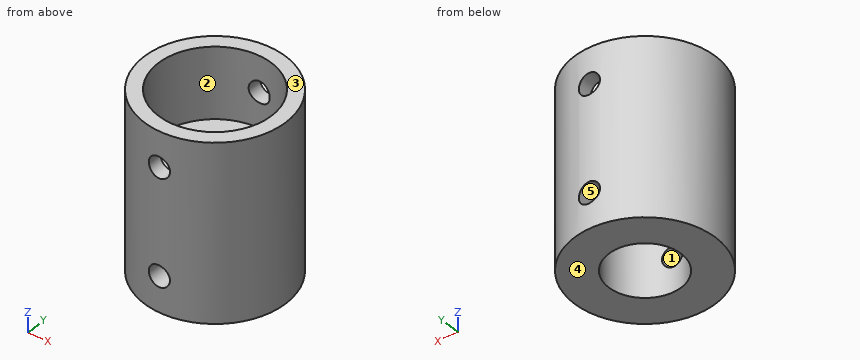
from build123d import *

# Parameters (mm, degrees)
ESQUISSE1_R                  = 20
ESQUISSE1_R_2                = 10.25
BOSS_EXTRU_1_DEPTH           = 50
ESQUISSE2_R                  = 16
ENL_V_MAT_EXTRU_1_DEPTH      = 20
ESQUISSE3_R                  = 3
ENL_V_MAT_EXTRU_2_DEPTH      = 21
ENL_V_MAT_EXTRU_2_DEPTH_BACK = 21


with BuildPart() as part:
    # Esquisse1 → Boss.-Extru.1 (new body)
    with BuildSketch(Plane.XY):
        Circle(ESQUISSE1_R)
        Circle(ESQUISSE1_R_2, mode=Mode.SUBTRACT)
    extrude(amount=BOSS_EXTRU_1_DEPTH)

    # Esquisse2 → Enlèv. mat.-Extru.1 (cut)
    with BuildSketch(Plane.XY.offset(50)):
        Circle(ESQUISSE2_R)
    extrude(amount=-ENL_V_MAT_EXTRU_1_DEPTH, mode=Mode.SUBTRACT)

    # Esquisse3 → Enlèv. mat.-Extru.2 (cut, two sides)
    with BuildSketch(Plane(origin=(0, 0, 0), x_dir=(1, 0, 0), z_dir=(0, 1, 0))) as enl_v_mat_extru_2_sk:
        with Locations(Location((0, -10, 0), (0, 0, 270))):  # turned: the seam where the file's is
            Circle(ESQUISSE3_R)
        with Locations(Location((0, -40, 0), (0, 0, 270))):  # turned: the seam where the file's is
            Circle(ESQUISSE3_R)
    extrude(amount=ENL_V_MAT_EXTRU_2_DEPTH, mode=Mode.SUBTRACT)
    extrude(enl_v_mat_extru_2_sk.sketch, amount=-ENL_V_MAT_EXTRU_2_DEPTH_BACK, mode=Mode.SUBTRACT)


solid = part.part
Geometry: final body of the model. Coordinates: model frame, mm. Face numbers are marked on the shaded views. A direction names the side the tool comes from. Coordinates: 2 decimals unless noted, no trailing zeros. Order: outer loops, then holes, each group sorted by start corner. A loop starts at its lowest first (then second) coordinate and runs counter-clockwise, first axis right, second up. Notation, with made-up numbers: M 16,36 L 59,36 A23 ccw 59,50 Z; hole C 13,4.5 d10. An arc over 180 degrees is marked long. One line per question, with ' | ' between items. Start each with the question number.
Item 1: Cut plane D-D, the plane z = 33. Return the cut outline in (x, y).
Item 2: Pin query (flat end, axial travel): pin 1 Ø8 at (x, z) = (-12, 18) entering from -Y; pin 2 Ø8 at (y, z) = (16, 35) entering from -X; pin 3 Ø5 at (y, z) = (14, 40) entering from -X. Return the tip coordinate at first contact, or that it passes through.
Item 3: Ray query, probe 1 along Z at (x, y) = (0, -17); probe 2 along Y at (x, z) = (0, 4); probe 3 along Z at (x, y) = (0, -15.75). Return the intervals inside material, ascending. Write a range as [from, to].
Item 4: Cut plane C-C, the plane z = 9. Return the cut outline in (x, y).
Item 5: Cut plane B-B, the plane y = 2. Return the cut outline in (x, z).
Item 6: Set-up query: the marked faces 1 and 2. Return all of +Z, -Z, +X, -X, +Y, -Y with unobstructed straight access to the full face (end or side cutting, diameter ignored); none if empty.
Item 7: Cut plane A-A, the plane x = 0. Return the cut outline in (y, z), then the cut area to 3 significant figures.
Item 8: Draft query along Z for the marked faces 3, 4 and 5. Return one class per face: released by +Z, released by -Z, zero draft, split by the parting line, or undercut.
A:
1) outline: C 0,0 d40; hole C 0,0 d32
2) pin 1: stops at y = -18.33 | pin 2: stops at x = -16 | pin 3: stops at x = -16.36
3) probe 1: z = [0, 7], [13, 37], [43, 50] | probe 2: y = [-20, -10.25], [10.25, 20] | probe 3: z = [0, 7], [13, 30]
4) outline: M -2.83,-19.8 L -2.83,-9.85 A10.25 cw -2.83,9.85 L -2.83,19.8 A20 ccw Z; M 2.83,-19.8 A20 ccw 2.83,19.8 L 2.83,9.85 A10.25 cw 2.83,-9.85 Z
5) outline: M -19.9,0 L -10.05,0 L -10.05,30 L -15.87,30 L -15.87,50 L -19.9,50 Z; M 10.05,0 L 19.9,0 L 19.9,50 L 15.87,50 L 15.87,30 L 10.05,30 Z
6) face 1: +Y, -Y | face 2: +Z
7) outline: M -20,0 L -10.25,0 L -10.25,7 L -20,7 Z; M -20,13 L -10.25,13 L -10.25,30 L -16,30 L -16,37 L -20,37 Z; M -20,43 L -16,43 L -16,50 L -20,50 Z; M 10.25,0 L 20,0 L 20,7 L 10.25,7 Z; M 10.25,13 L 20,13 L 20,37 L 16,37 L 16,30 L 10.25,30 Z; M 16,43 L 20,43 L 20,50 L 16,50 Z | area: 580 mm2
8) face 3: released by +Z | face 4: released by -Z | face 5: undercut
